Here's how the part is built. I have some questions about the finished solid (model axes, mm). Coordinates: 2 decimals unless noted, no trailing zeros. Write each loop counter-clockwise with the first axis right and the second up, starting at its lowest first coordinate (ties: lowest second). Pieces come first, ordered by that corner, then holes.
Item 1: I'm going to push flat-ended pins straight in: pin 1 Ø4.5 at (x, z) = (5.5, 74) entering from +Y; pin 2 Ø3 at (x, z) = (2, 174) entering from +Y. Where does each tip first touch, or does it pass through?
Item 2: If I drill on line 1 (Z direction, x = 3, y = -4.5); line 2 (Z direction, x = 6, y = -11.5); line 3 (Y direction, x = 3, z = 258), over which ranges is the centre line in solid material (lowest first)?
Item 3: If we section it at A-A (z = 265): Please give me the cut outline in (x, y).
Autodesk Fusion 360 part; units mm, degrees
sketch "Basic shape" plane through (0, 0, 0) normal (1, 0, 0) x (0, 0, -1)
  line L0 (0, 0) -> (-348.5, 0)
  line L1 (-348.5, 0) -> (-348.5, -48)
  line L2 (-348.5, -48) -> (0, -48)
  line L3 (0, -48) -> (0, 0)
  line L4 (-50, 0) -> (-99.5, 0)
  line L5 (-99.5, 0) -> (-99.5, -8)
  line L6 (-99.5, -8) -> (-50, -8)
  line L7 (-50, -8) -> (-50, 0)
  line L8 (-149.5, 0) -> (-199, 0)
  line L9 (-199, 0) -> (-199, -8)
  line L10 (-199, -8) -> (-149.5, -8)
  line L11 (-149.5, -8) -> (-149.5, 0)
  line L12 (-249, 0) -> (-298.5, 0)
  line L13 (-298.5, 0) -> (-298.5, -8)
  line L14 (-298.5, -8) -> (-249, -8)
  line L15 (-249, -8) -> (-249, 0)
  line L16 (-298.5, -8) -> (-348.5, -8) construction
  line L17 (-199, -8) -> (-249, -8) construction
  line L18 (-99.5, -8) -> (-149.5, -8) construction
  line L19 (-50, -8) -> (0, -8) construction
  dimension "d10" = 50
  dimension "d12" = 8
  dimension "d13" = 348.5
  dimension "d14" = 36.1667
  dimension "d246" = 40
extrude "Extrude1" add sketch "Basic shape" along normal blind 8 contours L0 L1 L2 L3 L5 L6 L7 L9 L10 L11 L13 L14 L15
sketch "T slots" plane through (0, 0, 0) normal (-1, 0, 0) x (0, 0, 1)
  line L0 (348.5, 0) -> (298.5, 0)
  line L1 (298.5, 0) -> (298.5, -8)
  line L2 (298.5, -8) -> (249, -8)
  line L3 (249, -8) -> (249, 0)
  line L4 (249, 0) -> (199, 0)
  line L5 (199, 0) -> (199, -8)
  line L6 (199, -8) -> (149.5, -8)
  line L7 (149.5, -8) -> (149.5, 0)
  line L8 (149.5, 0) -> (99.5, 0)
  line L9 (99.5, 0) -> (99.5, -8)
  line L10 (99.5, -8) -> (50, -8)
  line L11 (50, -8) -> (50, 0)
  line L12 (50, 0) -> (0, 0)
  line L13 (0, 0) -> (0, -48)
  line L14 (0, -48) -> (348.5, -48)
  line L15 (348.5, -48) -> (348.5, 0)
  line L16 (72.74, -8) -> (76.76, -8)
  line L17 (76.76, -8) -> (76.76, -25.5)
  line L18 (76.76, -25.5) -> (72.74, -25.5)
  line L19 (72.74, -25.5) -> (72.74, -8)
  line L20 (71.27, -13) -> (78.27, -13)
  line L21 (78.27, -13) -> (78.27, -20.5)
  line L22 (78.27, -20.5) -> (71.27, -20.5)
  line L23 (71.27, -20.5) -> (71.27, -13)
  line L24 (170.77, -20.5) -> (170.77, -13)
  line L25 (172.24, -8) -> (176.26, -8)
  line L26 (170.77, -13) -> (177.77, -13)
  line L27 (172.24, -25.5) -> (172.24, -8)
  line L28 (176.26, -8) -> (176.26, -25.5)
  line L29 (177.77, -20.5) -> (170.77, -20.5)
  line L30 (177.77, -13) -> (177.77, -20.5)
  line L31 (176.26, -25.5) -> (172.24, -25.5)
  line L32 (277.27, -20.5) -> (270.27, -20.5)
  line L33 (270.27, -13) -> (277.27, -13)
  line L34 (275.76, -8) -> (275.76, -25.5)
  line L35 (271.74, -25.5) -> (271.74, -8)
  line L36 (275.76, -25.5) -> (271.74, -25.5)
  line L37 (271.74, -8) -> (275.76, -8)
  line L38 (277.27, -13) -> (277.27, -20.5)
  line L39 (270.27, -20.5) -> (270.27, -13)
  circle A0 centre (275.27, -15) radius 2
  circle A1 centre (275.27, -18.5) radius 2
  dimension "d17" = 17.5
  dimension "d18" = 4.02
  dimension "d19" = 7
  dimension "d20" = 1.51
  dimension "d21" = 5
  dimension "d23" = 7.5
  dimension "d29" = 2.01
  dimension "d247" = 17.5
  dimension "d248" = 4.02
  dimension "d249" = 7
  dimension "d250" = 1.51
  dimension "d251" = 5
  dimension "d252" = 7.5
  dimension "d253" = 2.01
  dimension "d254" = 17.5
  dimension "d255" = 4.02
  dimension "d256" = 7
  dimension "d257" = 1.51
  dimension "d258" = 5
  dimension "d259" = 7.5
  dimension "d260" = 2.01
  dimension "d357" = 4
  dimension "d358" = 4
extrude "Extrude2" cut sketch "T slots" against normal through all contours L2 L33 L34 L35 L37 | L33 L34 A0 | L33 L34 L38 A0 | L32 L33 L35 L39 | L32 L33 L35 A0 A1 | L34 A0 A1 | L34 A0 A1 | L32 L34 L35 L36 | L34 A0 A1 | L34 A0 A1 | L38 A0 A1 | L34 A0 A1 | L10 L16 L17 L19 L20 | L32 L34 A1 | L34 A0 A1 | L32 L34 L38 A1 | L17 L19 L20 L22 | L19 L20 L22 L23 | L17 L20 L21 L22 | L17 L18 L19 L22 | L6 L25 L26 L27 L28 | L26 L27 L28 L29 | L26 L28 L29 L30 | L24 L26 L27 L29 | L27 L28 L29 L31
hole "Hole24" at (8, 1, 283.5) direction (-1, 0, 0) diameter 4 depth 10 tip angle 180
hole "Hole25" at (8, 1, 65) direction (-1, 0, 0) diameter 4 depth 10 tip angle 180
hole "Hole26" at (8, 1, 87.8333) direction (-1, 0, 0) diameter 4 depth 10 tip angle 180
hole "Hole27" at (8, 1, 185.6667) direction (-1, 0, 0) diameter 4 depth 10 tip angle 180
hole "Hole28" at (8, 1, 260.6667) direction (-1, 0, 0) diameter 4 depth 10 tip angle 180
hole "Hole29" at (8, 1, 162.8333) direction (-1, 0, 0) diameter 4 depth 10 tip angle 180
equation "d10 = Square_joint_thickness"
equation "pannel_thickness = 8 mm"
equation "d12 = pannel_thickness * 3 / 3"
equation "d15 = pannel_thickness"
equation "d20 = ( ( ( 7 - 4 ) / 2 ) * 1 mm ) + 0.01 mm"
equation "d250 = ( ( ( 7 - 4 ) / 2 ) * 1 mm ) + 0.01 mm"
equation "d257 = ( ( ( 7 - 4 ) / 2 ) * 1 mm ) + 0.01 mm"
equation "dbToolDia = 4 mm"
equation "dbOffset = 0 mm"
equation "dbRadius = ( dbToolDia + dbOffset ) / 2"
equation "dbHoleOffset = dbRadius / sqrt(2)"
equation "d530 = dbRadius * 2"
equation "d532 = dbHoleOffset"
equation "d533 = dbHoleOffset"
equation "d535 = dbRadius * 2"
equation "d537 = dbHoleOffset"
equation "d538 = dbHoleOffset"
equation "d540 = dbRadius * 2"
equation "d542 = dbHoleOffset"
equation "d543 = dbHoleOffset"
equation "d545 = dbRadius * 2"
equation "d547 = dbHoleOffset"
equation "d548 = dbHoleOffset"
equation "d550 = dbRadius * 2"
equation "d552 = dbHoleOffset"
equation "d553 = dbHoleOffset"
equation "d555 = dbRadius * 2"
equation "d557 = dbHoleOffset"
equation "d558 = dbHoleOffset"
equation "Square_joint_thickness = 50 mm"
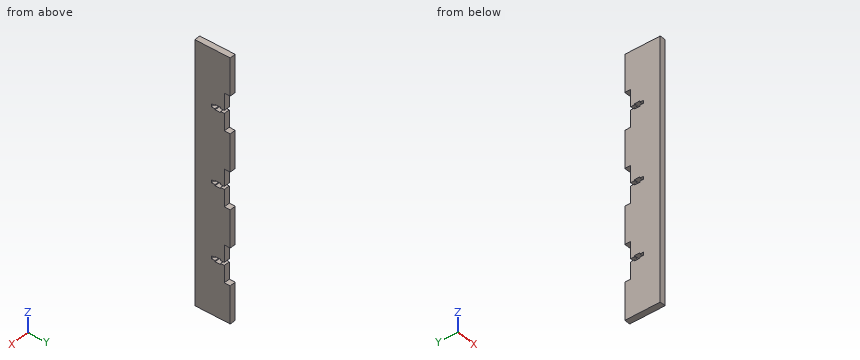
Answer list:
1. pin 1: stops at y = -8
1. pin 2: stops at y = -25.5
2. line 1: z = 0 to 50, 99.5 to 149.5, 199 to 249, 298.5 to 348.5
2. line 2: z = 0 to 72.74, 76.76 to 172.24, 176.26 to 271.74, 275.76 to 348.5
2. line 3: y = -48 to -8
3. outline: (0, -48) - (8, -48) - (8, -8) - (0, -8) - close
